```python
from build123d import *

# Parameters (mm, degrees)
SKETCH_1_R               = 15
EXTRUDE_3_DEPTH          = 30
SKETCH_4_R               = 5
EXTRUDE_4_DEPTH          = 5
SKETCH_5_R               = 5
EXTRUDE_5_DEPTH          = 5
FILLET_1_R               = 6
SKETCH_1_3_R             = 12.5
CUT_EXTRUDE_4_DEPTH      = 31
CUT_EXTRUDE_4_DEPTH_BACK = 31
CUT_EXTRUDE_3_REACH      = 38.213


with BuildPart() as part:
    # 草圖1 → 填料-伸長3 (new body, symmetric)
    with BuildSketch(Plane(origin=(0, 0, 0), x_dir=(1, 0, 0), z_dir=(0, 1, 0))):
        Circle(SKETCH_1_R)
    extrude(amount=EXTRUDE_3_DEPTH, both=True)

    # 草圖4 → 填料-伸長4 (add)
    with BuildSketch(Plane.ZY.offset(15)):
        with BuildLine():
            Line((0, -17.5), (0, 17.5))
            Line((0, 17.5), (32.338287195, 9.722778049))
            ThreePointArc((32.338287195, 9.722778049), (40, 0), (32.338287195, -9.722778049))
            Line((32.338287195, -9.722778049), (0, -17.5))
        make_face()
        with Locations((30, 0)):
            Circle(SKETCH_4_R, mode=Mode.SUBTRACT)
    extrude(amount=-EXTRUDE_4_DEPTH)

    # 草圖5 → 填料-伸長5 (add)
    with BuildSketch(Plane(origin=(0, 0, -15), x_dir=(-1, 0, 0), z_dir=(0, 0, -1))):
        with BuildLine():
            Line((0, -17.5), (0, 17.5))
            Line((0, 17.5), (-32.338287195, 9.722778049))
            ThreePointArc((-32.338287195, 9.722778049), (-40, 0), (-32.338287195, -9.722778049))
            Line((-32.338287195, -9.722778049), (0, -17.5))
        make_face()
        with Locations((-30, 0)):
            Circle(SKETCH_5_R, mode=Mode.SUBTRACT)
    extrude(amount=-EXTRUDE_5_DEPTH)

    # 圓角1
    fillet_1_edges = [part.edges().sort_by_distance(p)[0] for p in [
        (11.180339887, 0, -10),
        (-10, 0, 11.180339887),
    ]]
    fillet(fillet_1_edges, radius=FILLET_1_R)

    # 草圖1<3> → 除料-伸長4 (cut, two sides)
    with BuildSketch(Plane(origin=(0, 0, 0), x_dir=(1, 0, 0), z_dir=(0, 1, 0))) as cut_extrude_4_sk:
        Circle(SKETCH_1_3_R)
    extrude(amount=CUT_EXTRUDE_4_DEPTH, mode=Mode.SUBTRACT)
    extrude(cut_extrude_4_sk.sketch, amount=-CUT_EXTRUDE_4_DEPTH_BACK, mode=Mode.SUBTRACT)

    # 草圖7 → 除料-伸長3 (cut, up to next)
    with BuildSketch(Plane(origin=(10.606601718, 0, 10.606601718), x_dir=(0.707106781, 0, -0.707106781), z_dir=(0.707106781, 0, 0.707106781)), mode=Mode.PRIVATE) as cut_extrude_3_sk1:
        with BuildLine():
            Line((-7, 25), (7, 25))
            ThreePointArc((7, 25), (9.121320344, 24.121320344), (10, 22))
            Line((10, 22), (10, 8))
            ThreePointArc((10, 8), (9.121320344, 5.878679656), (7, 5))
            Line((7, 5), (-7, 5))
            ThreePointArc((-7, 5), (-9.121320344, 5.878679656), (-10, 8))
            Line((-10, 8), (-10, 22))
            ThreePointArc((-10, 22), (-9.121320344, 24.121320344), (-7, 25))
        make_face()
    cut_extrude_3_tool1 = extrude(cut_extrude_3_sk1.sketch, amount=-CUT_EXTRUDE_3_REACH, mode=Mode.PRIVATE) & part.part
    add(cut_extrude_3_tool1.solids().sort_by_distance((10.606602, 15, 10.606602))[0], mode=Mode.SUBTRACT)
    # 草圖7 → 除料-伸長3 (cut, up to next)
    with BuildSketch(Plane(origin=(10.606601718, 0, 10.606601718), x_dir=(0.707106781, 0, -0.707106781), z_dir=(0.707106781, 0, 0.707106781)), mode=Mode.PRIVATE) as cut_extrude_3_sk2:
        with BuildLine():
            Line((-7, -5), (7, -5))
            ThreePointArc((7, -5), (9.121320344, -5.878679656), (10, -8))
            Line((10, -8), (10, -22))
            ThreePointArc((10, -22), (9.121320344, -24.121320344), (7, -25))
            Line((7, -25), (-7, -25))
            ThreePointArc((-7, -25), (-9.121320344, -24.121320344), (-10, -22))
            Line((-10, -22), (-10, -8))
            ThreePointArc((-10, -8), (-9.121320344, -5.878679656), (-7, -5))
        make_face()
    cut_extrude_3_tool2 = extrude(cut_extrude_3_sk2.sketch, amount=-CUT_EXTRUDE_3_REACH, mode=Mode.PRIVATE) & part.part
    add(cut_extrude_3_tool2.solids().sort_by_distance((10.606602, -15, 10.606602))[0], mode=Mode.SUBTRACT)


solid = part.part
```
Geometry check sheet. Reference: the model listing, model coordinates, mm. A direction names the side the tool comes from. Round coordinates to 2 decimals unless told otherwise and drop trailing zeros. Loops run counter-clockwise (first coordinate to the right, second up) from the corner with the lowest first, then second, coordinate; pieces in that order, holes last. Notation, with made-up numbers: (74.5, -27) -> (88.5, -27) arc R19 ccw to (88.5, 0) -> close; hole circle Ø11 at (5, 47.5). An arc over 180 degrees is marked (long way). Use a Markdown table: item, result.
(1) Sectioned sample at C-C (x = 10). Enter the section's corners in (y, z), then the cut area to 3 significant figures.
Calculated:
| item | result |
|---|---|
| outline | (-30, -11.18) -> (-15.1, -11.18) -> (-15.1, -15) -> (15.1, -15) -> (15.1, -11.18) -> (30, -11.18) -> (30, -7.5) -> (-30, -7.5) -> close; (-30, 7.5) -> (-25, 7.5) -> (-25, 11.18) -> (-30, 11.18) -> close; (-5, 7.5) -> (5, 7.5) -> (5, 11.18) -> (-5, 11.18) -> close; (25, 7.5) -> (30, 7.5) -> (30, 11.18) -> (25, 11.18) -> close |
| area | 410 mm² |
(2) Sectioned sample at A-A (z = 29). Enter the section's corners in (x, y).
Calculated:
| item | result |
|---|---|
| outline | (-15, -10.53) -> (-10, -10.53) -> (-10, -4.9) -> (-15, -4.9) -> close; (-15, 4.9) -> (-10, 4.9) -> (-10, 10.53) -> (-15, 10.53) -> close |
(3) Set-up check for faces 1 (the cylindrical face through (13.837, 5.902, 0.904)), 2 (the cylindrical face through (0.904, 24.098, 13.837)), 3 (the cylindrical face through (-11.056, 0.42, -10.138)), 4 (the flat face through (-10, 0, 24)): record each of +Z, -Z, +X, -X, +Y, -Y from which the full face is reachable in a straight line by a thin tool's end or side.
Calculated:
| item | result |
|---|---|
| face 1 | +Z |
| face 2 | +X |
| face 3 | none |
| face 4 | +Z, +X, +Y, -Y |
(4) Sectioned sample at D-D (z = 9). Enter the section's corners in (x, y), then the cut area to 3 significant figures.
Calculated:
| item | result |
|---|---|
| outline | (-15, -15.34) -> (-12, -15.34) -> (-12, -30) -> (-8.67, -30) -> (-8.67, 30) -> (-12, 30) -> (-12, 15.34) -> (-15, 15.34) -> close; (8.67, -30) -> (12, -30) -> (12, -25) -> (8.67, -25) -> close; (8.67, -5) -> (12, -5) -> (12, 5) -> (8.67, 5) -> close; (8.67, 25) -> (12, 25) -> (12, 30) -> (8.67, 30) -> close |
| area | 358 mm² |
(5) Go/stop test with flat-tipped pins: P1, Ø16, axis at y = 0, z = 30, coming from the -X side; P2, Ø6, axis at y = -0.5, z = 33, coming from the +X side; P3, Ø8, axis at x = 34.5, y = -5.5, coming from the +Z side; P4, Ø21.5, axis at x = 28, y = 0, coming from the +Z side. Record where each tip stops, or that it passes through.
Calculated:
| item | result |
|---|---|
| P1 | x = -15 |
| P2 | x = -10 |
| P3 | z = -10 |
| P4 | z = -8.97 |
(6) Scan lines: probe 1 along X at (y, z) = (-2.5, 0); probe 2 along X at (y, z) = (-3.5, 11); probe 3 along Z at (x, y) = (-11.5, 4.5). Record each from-to range of solid material in increasing order.
Calculated:
| item | result |
|---|---|
| probe 1 | -15 to -12.5, 12.5 to 15 |
| probe 2 | -15 to -5.94, 5.94 to 10.2 |
| probe 3 | -9.63 to -4.9, 4.9 to 27.82, 32.18 to 38.93 |
(7) Mould release check, pull along X, two halves, no side actions. Record for faces 5 (the cylindrical face through (13.804, -5.855, 0.937)), 6 (the flat face through (-0.45, 14.9, 13.69)), 7 (the flat face through (-15, 0, 16)): released by +X, released by -X, zero draft, split by the parting line, or undercut.
Calculated:
| item | result |
|---|---|
| face 5 | undercut |
| face 6 | released by +X |
| face 7 | released by -X |
(8) Sectioned sample at B-B (x = 30). Enter the section's corners in (y, z).
Calculated:
| item | result |
|---|---|
| outline | (-10.29, -15) -> (-5, -15) -> (-5, -10) -> (-10.29, -10) -> close; (5, -15) -> (10.29, -15) -> (10.29, -10) -> (5, -10) -> close |
